Verification items for the finished model (mm, model axes). A direction names the side the tool comes from. Coordinates: 2 decimals unless noted, no trailing zeros. Write each loop counter-clockwise with the first axis right and the second up, starting at its lowest first coordinate (ties: lowest second). Pieces come first, ordered by that corner, then holes. Notation, with made-up numbers: (-35, -7.5) -> (-16, -7.5) arc R37 cw to (-16, 28.5) -> close; hole circle Ø1 at (-36.75, 87.25). An arc over 180 degrees is marked (long way). Answer in a Markdown table with one row per item.
```python
from build123d import *

# Parameters (mm, degrees)
SKETCH1_R           = 6.35
BOSS_EXTRUDE2_DEPTH = 12.7


with BuildPart() as part:
    # Sketch1 → Boss-Extrude2 (new body)
    with BuildSketch(Plane.XY):
        with BuildLine():
            Line((-12.031647615, 4.065643329), (-97.612603668, -249.198064906))
            ThreePointArc((-97.612603668, -249.198064906), (-98.010291731, -255.396978352), (-95.255242973, -260.964238904))
            Line((-95.255242973, -260.964238904), (-66.174198568, -294.032435491))
            ThreePointArc((-66.174198568, -294.032435491), (-63.209942623, -302.725331079), (-67.260702561, -310.968181978))
            Line((-67.260702561, -310.968181978), (-91.628287065, -332.397678599))
            ThreePointArc((-91.628287065, -332.397678599), (-92.778170458, -350.321343631), (-74.854505426, -351.471227024))
            Line((-74.854505426, -351.471227024), (-50.486920922, -330.041730403))
            ThreePointArc((-50.486920922, -330.041730403), (-41.794025334, -327.077474458), (-33.551174435, -331.128234397))
            Line((-33.551174435, -331.128234397), (-9.579195164, -358.386888249))
            ThreePointArc((-9.579195164, -358.386888249), (8.344469868, -359.536771642), (9.494353261, -341.61310661))
            Line((9.494353261, -341.61310661), (-14.47762601, -314.354452758))
            ThreePointArc((-14.47762601, -314.354452758), (-17.441881955, -305.66155717), (-13.391122016, -297.418706271))
            Line((-13.391122016, -297.418706271), (-12.865473044, -296.956436698))
            ThreePointArc((-12.865473044, -296.956436698), (-11.715589651, -279.032771666), (-29.639254683, -277.882888273))
            Line((-29.639254683, -277.882888273), (-30.164903655, -278.345157846))
            ThreePointArc((-30.164903655, -278.345157846), (-38.857799244, -281.309413791), (-47.100650142, -277.258653852))
            Line((-47.100650142, -277.258653852), (-66.497347204, -255.202575583))
            ThreePointArc((-66.497347204, -255.202575583), (-69.252395961, -249.635315031), (-68.854707898, -243.436401585))
            Line((-68.854707898, -243.436401585), (12.031647615, -4.065643329))
            ThreePointArc((12.031647615, -4.065643329), (4.065643329, 12.031647615), (-12.031647615, 4.065643329))
        make_face()
        with Locations((-21.252363864, -287.419662486)):
            Circle(SKETCH1_R, mode=Mode.SUBTRACT)
        with Locations((-83.241396246, -341.934452812)):
            Circle(SKETCH1_R, mode=Mode.SUBTRACT)
        with Locations((-0.042420952, -349.999997429)):
            Circle(SKETCH1_R, mode=Mode.SUBTRACT)
        Circle(SKETCH1_R, mode=Mode.SUBTRACT)
    extrude(amount=BOSS_EXTRUDE2_DEPTH)


solid = part.part
```
1. Go/stop test with flat-tipped pins: pin 1 (1.5 mm diameter, centred on x = -4, z = 9.5, fed in from -Y); pin 2 (1.5 mm diameter, centred on y = -142, z = 6.5, fed in from +X). Record where each tip stops, or that it passes through.
Findings below:
| item | result |
|---|---|
| pin 1 | stops at y = -362.29 |
| pin 2 | stops at x = -34.32 |
2. Access from +Z, -Z, +X, -X, +Y, -Y to the whole of each face (thin tool, end or side, straight path). Record for faces 4 (the face through (-28.98, -125.43, 6.26)), 5 (the face through (-98.027, -255.311, 6.261)), 6 (the face through (-21.73, -344.57, 6.26)).
Findings below:
| item | result |
|---|---|
| face 4 | +Z, -Z, +X |
| face 5 | +Z, -Z, -X |
| face 6 | +Z, -Z, -Y |
3. Material ranges on probe 1 along X at (y, z) = (-296.5, 7.25); probe 2 along X at (y, z) = (-55, 0.5), recorded low to high. Write a range as from..to.
Findings below:
| item | result |
|---|---|
| probe 1 | x = -64.5..-12.37 |
| probe 2 | x = -31.99..-5.18 |
4. Sectioned sample at D-D, the plane x = -38.5. Record the cut outline in (y, z).
Findings below:
| item | result |
|---|---|
| outline | (-327.76, 0) -> (-281.33, 0) -> (-281.33, 12.7) -> (-327.76, 12.7) -> close; (-153.61, 0) -> (-74.26, 0) -> (-74.26, 12.7) -> (-153.61, 12.7) -> close |
5. Release check for a two-part mould opening along Y. For faces 1 (the face through (-1.38, -6.2, 6.26)), 2 (the face through (-54.22, -120.79, 6.26)), 3 (the face through (-51, -188, 12.7)) record: released by +Y, released by -Y, zero draft, split by the parting line, or undercut.
Findings below:
| item | result |
|---|---|
| face 1 | undercut |
| face 2 | released by +Y |
| face 3 | zero draft |
6. Sectioned sample at B-B, the plane x = 0. Record the cut outline in (y, z).
Findings below:
| item | result |
|---|---|
| outline | (-362.7, 0) -> (-356.35, 0) -> (-356.35, 12.7) -> (-362.7, 12.7) -> close; (-343.65, 0) -> (-330.82, 0) -> (-330.82, 12.7) -> (-343.65, 12.7) -> close; (-39.67, 0) -> (-6.35, 0) -> (-6.35, 12.7) -> (-39.67, 12.7) -> close; (6.35, 0) -> (12.7, 0) -> (12.7, 12.7) -> (6.35, 12.7) -> close |
7. Sectioned sample at C-C, the plane z = 3.25. Record the cut outline in (x, y).
Findings below:
| item | result |
|---|---|
| outline | (-97.61, -249.2) arc R12 ccw to (-95.26, -260.96) -> (-66.17, -294.03) arc R12 cw to (-67.26, -310.97) -> (-91.63, -332.4) arc R12.7 ccw to (-74.85, -351.47) -> (-50.49, -330.04) arc R12 cw to (-33.55, -331.13) -> (-9.58, -358.39) arc R12.7 ccw to (9.49, -341.61) -> (-14.48, -314.35) arc R12 cw to (-13.39, -297.42) -> (-12.87, -296.96) arc R12.7 ccw to (-29.64, -277.88) -> (-30.16, -278.35) arc R12 cw to (-47.1, -277.26) -> (-66.5, -255.2) arc R12 cw to (-68.85, -243.44) -> (12.03, -4.07) arc R12.7 ccw to (-12.03, 4.07) -> close; hole circle Ø12.7 at (-83.24, -341.93); hole circle Ø12.7 at (-21.25, -287.42); hole circle Ø12.7 at (-0.04, -350); hole circle Ø12.7 at (0, 0) |
8. Sectioned sample at A-A, the plane y = 0. Record the cut outline in (x, z).
Findings below:
| item | result |
|---|---|
| outline | (-13.41, 0) -> (-6.35, 0) -> (-6.35, 12.7) -> (-13.41, 12.7) -> close; (6.35, 0) -> (12.7, 0) -> (12.7, 12.7) -> (6.35, 12.7) -> close |
